```python
from build123d import *

# Parameters (mm, degrees)
F1_DEPTH = 5
F3_D     = 5
F4_DEPTH = 7.5
F5_W     = 10
F5_H     = 4
F6_DEPTH = 2.5
F7_W     = 10
F7_H     = 4
F8_DEPTH = 2.5


with BuildPart() as f1:
    # F0 (on Right) → F1 (new body)
    with BuildSketch(Plane.YZ):
        with BuildLine():
            Line((-57.2294044495, 42.7520807087), (-57.2294044495, 37.7520807087))
            ThreePointArc((-57.2294044495, 37.7520807087), (-52.2294044495, 32.7520807087), (-47.2294044495, 37.7520807087))
            Line((-47.2294044495, 37.7520807087), (-47.2294044495, 42.7520807087))
            Line((-47.2294044495, 42.7520807087), (-57.2294044495, 42.7520807087))
        make_face()
    extrude(amount=F1_DEPTH)

    # F3 (through all)
    with Locations(Plane(origin=(0, 0, 0), x_dir=(0, -1, 0), z_dir=(-1, 0, 0))):
        with Locations((52.2294044495, 37.7520807087)):
            Hole(F3_D / 2)

    # F4 (add): a face of the model
    f4_faces = [f1.faces().sort_by_distance(p)[0] for p in [
        (2.5, -52.2294044495, 42.7520807087),
    ]]
    extrude(f4_faces, amount=F4_DEPTH)

    # F5 (on face) → F6 (join)
    with BuildSketch(Plane(origin=(0, 0, 0), x_dir=(0, -1, 0), z_dir=(-1, 0, 0))):
        with Locations((52.2294044495, 48.2520807087)):
            Rectangle(F5_W, F5_H)
    extrude(amount=F6_DEPTH)

    # F7 (on face) → F8 (join)
    with BuildSketch(Plane.YZ.offset(5)):
        with Locations((-52.2294044495, 48.2520807087)):
            Rectangle(F7_W, F7_H)
    extrude(amount=F8_DEPTH)


solid = f1.part
```
Input: part model. Units: mm. Frame: model coordinates. A direction names the side the tool comes from. Coordinates: 2 decimals unless noted, no trailing zeros. Loops run counter-clockwise (first coordinate to the right, second up) from the corner with the lowest first, then second, coordinate; pieces in that order, holes last. Notation, with made-up numbers: M 28.25,-23.5 L 49.25,-23.5 A14 cw 49.25,-19.5 Z; hole C 23.25,58.5 d6. An arc over 180 degrees is marked long. Answer in a Markdown table with one row per item.
1. First-contact query: pin 1 (6 mm diameter, centred on x = 1, y = -48.5, fed in from -Z); pin 2 (4 mm diameter, centred on y = -52.23, z = 37.75, fed in from -X); pin 3 (2 mm diameter, centred on y = -55.5, z = 34.5, fed in from +X); pin 4 (1.2 mm diameter, centred on x = -1, y = -49.5, fed in from -Z). Flat tips, straight axial feed; report the tip coordinate or a pass-through.
Response:
| item | result |
|---|---|
| pin 1 | stops at z = 32.81 |
| pin 2 | passes through |
| pin 3 | stops at x = 5 |
| pin 4 | stops at z = 46.25 |
2. Section B-B, the plane x = 2.75. Output: boundary loops of the cut face in (y, z).
Response:
| item | result |
|---|---|
| outline | M -57.23,37.75 A5 ccw -47.23,37.75 L -47.23,50.25 L -57.23,50.25 Z; hole C -52.23,37.75 d5 |
3. Reachability of faces 1 (the flat face through (5, -52, 41)), 2 (the flat face through (-2.5, -52, 48)), 3 (the flat face through (-1, -52, 46.252)) from +Z, -Z, +X, -X, +Y, -Y: full face, straight path, thin tool, end or side. Return the list, or none.
Response:
| item | result |
|---|---|
| face 1 | -Z, +X, +Y, -Y |
| face 2 | +Z, -Z, -X, +Y, -Y |
| face 3 | -Z, -X, +Y, -Y |
4. Draft query along Y for faces 4 (the cylindrical face through (2.535, -54.727, 37.862)), 5 (the cylindrical face through (2.465, -52.339, 32.753)), 6 (the flat face through (2, -57.229, 45)), 7 (the flat face through (0, -52, 41)). Return one class per face: pulls with the +Y half, pulls with the -Y half, needs draft (parallel to the pull), parting line crosses it, or undercut.
Response:
| item | result |
|---|---|
| face 4 | undercut |
| face 5 | parting line crosses it |
| face 6 | pulls with the -Y half |
| face 7 | needs draft |
5. Section D-D, the plane y = -52. Output: boundary loops of the cut face in (x, z), then the cut area to 3 significant figures.
Response:
| item | result |
|---|---|
| outline | M -2.5,46.25 L 0,46.25 L 0,40.24 L 5,40.24 L 5,46.25 L 7.5,46.25 L 7.5,50.25 L -2.5,50.25 Z; M 0,32.76 L 5,32.76 L 5,35.26 L 0,35.26 Z |
| area | 82.6 mm2 |
6. Material intervals for line 1 (Z direction, x = -0.5, y = -55.25); line 2 (X direction, y = -56, z = 44); line 3 (Z direction, x = 1, y = -54.5), sorted ascending.
Response:
| item | result |
|---|---|
| line 1 | z = 46.25 to 50.25 |
| line 2 | x = 0 to 5 |
| line 3 | z = 33.3 to 36.71, 38.8 to 50.25 |
7. Section A-A, the plane y = -54.25. Output: boundary loops of the cut face in (x, z), then the cut area to 3 significant figures.
Response:
| item | result |
|---|---|
| outline | M -2.5,46.25 L 0,46.25 L 0,39.22 L 5,39.22 L 5,46.25 L 7.5,46.25 L 7.5,50.25 L -2.5,50.25 Z; M 0,33.18 L 5,33.18 L 5,36.28 L 0,36.28 Z |
| area | 90.6 mm2 |
8. Section C-C, the plane x = -0.5. Output: boundary loops of the cut face in (y, z).
Response:
| item | result |
|---|---|
| outline | M -57.23,46.25 L -47.23,46.25 L -47.23,50.25 L -57.23,50.25 Z |
